from build123d import *

# Parameters (mm, degrees)
SKETCH1_R            = 2.75
SKETCH1_W            = 40
SKETCH1_H            = 15
BOSS_EXTRUDE1_DEPTH  = 10
SKETCH3_W            = 40
SKETCH3_H            = 5
BOSS_EXTRUDE2_DEPTH  = 43
CUT_EXTRUDE1_REACH   = 166.968
SKETCH4_R            = 1.75
SKETCH4_R_2          = 11
SKETCH8_W            = 4
SKETCH8_H            = 45
BOSS_EXTRUDE4_DEPTH  = 43
SKETCH11_W           = 40
SKETCH11_H           = 40
BOSS_EXTRUDE15_DEPTH = 3
FILLET3_R            = 1
FILLET6_R            = 1
FILLET7_R            = 1


with BuildPart() as part:
    # Sketch1 → Boss-Extrude1 (new body)
    with BuildSketch(Plane(origin=(0, 0, 0), x_dir=(1, 0, 0), z_dir=(0, 1, 0))):
        Polygon((51, 62.5), (51, 83.65), (99, 83.65), (99, 62.5), (150, 62.5), (150, 0), (0, 0), (0, 62.5), align=None)
        with Locations(Location((108.05464, 46, 0), (0, 0, 270))):
            Circle(SKETCH1_R, mode=Mode.SUBTRACT)
        with Locations(Location((41.87366, 46, 0), (0, 0, 270))):
            Circle(SKETCH1_R, mode=Mode.SUBTRACT)
        with Locations(Location((41.87366, 16.5, 0), (0, 0, 270))):
            Circle(SKETCH1_R, mode=Mode.SUBTRACT)
        with Locations(Location((108.05464, 16.5, 0), (0, 0, 270))):
            Circle(SKETCH1_R, mode=Mode.SUBTRACT)
        with Locations((75, 31.15)):
            Rectangle(SKETCH1_W, SKETCH1_H, mode=Mode.SUBTRACT)
    extrude(amount=BOSS_EXTRUDE1_DEPTH)

    # Sketch3 → Boss-Extrude2 (add)
    with BuildSketch(Plane(origin=(0, 10, 0), x_dir=(1, 0, 0), z_dir=(0, 1, 0))):
        with Locations((75, 41.15)):
            Rectangle(SKETCH3_W, SKETCH3_H)
    extrude(amount=BOSS_EXTRUDE2_DEPTH)

    # Sketch4 → Cut-Extrude1 (cut, up to next)
    with BuildSketch(Plane(origin=(0, 0, -43.65), x_dir=(-1, 0, 0), z_dir=(0, 0, -1)), mode=Mode.PRIVATE) as cut_extrude1_sk1:
        with Locations((-59.5, 18.25)):
            Circle(SKETCH4_R)
    cut_extrude1_tool1 = extrude(cut_extrude1_sk1.sketch, amount=-CUT_EXTRUDE1_REACH, mode=Mode.PRIVATE) & part.part
    # Sketch4 → Cut-Extrude1 (cut, up to next)
    with BuildSketch(Plane(origin=(0, 0, -43.65), x_dir=(-1, 0, 0), z_dir=(0, 0, -1)), mode=Mode.PRIVATE) as cut_extrude1_sk2:
        with Locations((-90.5, 18.25)):
            Circle(SKETCH4_R)
    cut_extrude1_tool2 = extrude(cut_extrude1_sk2.sketch, amount=-CUT_EXTRUDE1_REACH, mode=Mode.PRIVATE) & part.part
    # Sketch4 → Cut-Extrude1 (cut, up to next)
    with BuildSketch(Plane(origin=(0, 0, -43.65), x_dir=(-1, 0, 0), z_dir=(0, 0, -1)), mode=Mode.PRIVATE) as cut_extrude1_sk3:
        with Locations((-75, 33.75)):
            Circle(SKETCH4_R_2)
    cut_extrude1_tool3 = extrude(cut_extrude1_sk3.sketch, amount=-CUT_EXTRUDE1_REACH, mode=Mode.PRIVATE) & part.part
    # Sketch4 → Cut-Extrude1 (cut, up to next)
    with BuildSketch(Plane(origin=(0, 0, -43.65), x_dir=(-1, 0, 0), z_dir=(0, 0, -1)), mode=Mode.PRIVATE) as cut_extrude1_sk4:
        with Locations((-90.5, 49.25)):
            Circle(SKETCH4_R)
    cut_extrude1_tool4 = extrude(cut_extrude1_sk4.sketch, amount=-CUT_EXTRUDE1_REACH, mode=Mode.PRIVATE) & part.part
    # Sketch4 → Cut-Extrude1 (cut, up to next)
    with BuildSketch(Plane(origin=(0, 0, -43.65), x_dir=(-1, 0, 0), z_dir=(0, 0, -1)), mode=Mode.PRIVATE) as cut_extrude1_sk5:
        with Locations((-59.5, 49.25)):
            Circle(SKETCH4_R)
    cut_extrude1_tool5 = extrude(cut_extrude1_sk5.sketch, amount=-CUT_EXTRUDE1_REACH, mode=Mode.PRIVATE) & part.part
    add(cut_extrude1_tool1.solids().sort_by_distance((59.5, 18.25, -43.65))[0], mode=Mode.SUBTRACT)
    add(cut_extrude1_tool2.solids().sort_by_distance((90.5, 18.25, -43.65))[0], mode=Mode.SUBTRACT)
    add(cut_extrude1_tool3.solids().sort_by_distance((75, 33.75, -43.65))[0], mode=Mode.SUBTRACT)
    add(cut_extrude1_tool4.solids().sort_by_distance((90.5, 49.25, -43.65))[0], mode=Mode.SUBTRACT)
    add(cut_extrude1_tool5.solids().sort_by_distance((59.5, 49.25, -43.65))[0], mode=Mode.SUBTRACT)

    # Sketch8 → Boss-Extrude4 (add)
    with BuildSketch(Plane(origin=(0, 10, 0), x_dir=(1, 0, 0), z_dir=(0, 1, 0))):
        with Locations((53, 61.15)):
            Rectangle(SKETCH8_W, SKETCH8_H)
        with Locations((97, 61.15)):
            Rectangle(SKETCH8_W, SKETCH8_H)
    extrude(amount=BOSS_EXTRUDE4_DEPTH)

    # Sketch11 → Boss-Extrude15 (add)
    with BuildSketch(Plane(origin=(0, 10, 0), x_dir=(1, 0, 0), z_dir=(0, 1, 0))):
        with Locations((75, 63.65)):
            Rectangle(SKETCH11_W, SKETCH11_H)
    extrude(amount=BOSS_EXTRUDE15_DEPTH)

    # Fillet3
    fillet3_edges = [part.edges().sort_by_distance(p)[0] for p in [
        (55, 0, -31.15),
        (75, 0, -23.65),
        (95, 0, -31.15),
        (75, 0, -38.65),
        (55, 5, -38.65),
        (55, 5, -23.65),
        (95, 5, -23.65),
        (95, 5, -38.65),
    ]]
    fillet(fillet3_edges, radius=FILLET3_R)

    # Fillet6
    fillet6_edges = [part.edges().sort_by_distance(p)[0] for p in [
        (99, 10, -50.575),
        (51, 10, -50.575),
    ]]
    fillet(fillet6_edges, radius=FILLET6_R)

    # Fillet7
    fillet7_edges = [part.edges().sort_by_distance(p)[0] for p in [
        (99, 5.5, -62.5),
        (51, 5.5, -62.5),
    ]]
    fillet(fillet7_edges, radius=FILLET7_R)


solid = part.part
Input: part model. Units: mm. Frame: model coordinates. A direction names the side the tool comes from. Give positions to 0.01 mm unless a question says otherwise; leave off trailing zeros. Order: outer loops, then holes, each group sorted by start corner. A loop starts at its lowest first (then second) coordinate and runs counter-clockwise, first axis right, second up.
Q1. Section A-A on y = 49.25. Output: boundary loops of the cut face in (x, z), and give its area (3 significant figures).
Checked values:
outline: (51, -83.65) - (55, -83.65) - (55, -43.65) - (57.75, -43.65) - (57.75, -38.65) - (51, -38.65) - close; (61.25, -43.65) - (88.75, -43.65) - (88.75, -38.65) - (61.25, -38.65) - close; (92.25, -43.65) - (95, -43.65) - (95, -83.65) - (99, -83.65) - (99, -38.65) - (92.25, -38.65) - close
area: 525 mm2
Q2. Section C-C on x = 90.5. Output: boundary loops of the cut face in (y, z).
Checked values:
outline: (0, -83.65) - (13, -83.65) - (13, -43.65) - (16.5, -43.65) - (16.5, -38.65) - (1, -38.65) arc R1 ccw to (0, -39.65) - close; (0, -22.65) arc R1 ccw to (1, -23.65) - (10, -23.65) - (10, 0) - (0, 0) - close; (20, -43.65) - (47.5, -43.65) - (47.5, -38.65) - (20, -38.65) - close; (51, -43.65) - (53, -43.65) - (53, -38.65) - (51, -38.65) - close
Q3. Contact query for flat-ended pins moving along their axis: pin 1 Ø2 at (y, z) = (14.5, -65) entering from +X; pin 2 Ø1 at (x, z) = (25, -55.5) entering from +Y; pin 3 Ø5 at (x, y) = (132, 3.5) entering from -Z. Output: stop coordinate, or through.
Checked values:
pin 1: stops at x = 99
pin 2: stops at y = 10
pin 3: stops at z = -62.5
Q4. Draft query along X for faces 4 (the cylindrical face through (105.37, 4.93, -17.1)), 5 (the flat face through (51, 26, -61)), 6 (the flat face through (76, 5, 0)). Return one class per face: +X half, -X half, draft (parallel to the pull), parting line (faces both ways), or undercut.
Checked values:
face 4: undercut
face 5: -X half
face 6: draft
Q5. Set-up query: faces 1 (the flat face through (95, 5, -31)), 2 (the flat face through (66, 24, -43.65)), 3 (the flat face through (76, 10, -18)). Return all of +Z, -Z, +X, -X, +Y, -Y with unobstructed straight access to the full face (end or side cutting, diameter ignored); none if empty.
Checked values:
face 1: +Y, -Y
face 2: -Z, +Y
face 3: +Z, +Y
Q6. Ray query, probe 1 along X at (y, z) = (2.5, -46); probe 2 along X at (y, z) = (18, -41); probe 3 along Y at (x, z) = (59.5, -39.75). Return the intervals inside material, ascending.
Checked values:
probe 1: x = 0 to 39.12, 44.62 to 105.3, 110.8 to 150
probe 2: x = 51 to 57.77, 61.23 to 88.77, 92.23 to 99
probe 3: y = 0 to 16.5, 20 to 47.5, 51 to 53
Q7. Section D-D on x = 75. Output: boundary loops of the cut face in (y, z), and give its area (3 significant figures).
Checked values:
outline: (0, -83.65) - (13, -83.65) - (13, -43.65) - (22.75, -43.65) - (22.75, -38.65) - (1, -38.65) arc R1 ccw to (0, -39.65) - close; (0, -22.65) arc R1 ccw to (1, -23.65) - (10, -23.65) - (10, 0) - (0, 0) - close; (44.75, -43.65) - (53, -43.65) - (53, -38.65) - (44.75, -38.65) - close
area: 911 mm2
Q8. Section B-B on z = -16.5. Output: boundary loops of the cut face in (x, y), and give its area (3 significant figures).
Checked values:
outline: (0, 0) - (39.12, 0) - (39.12, 10) - (0, 10) - close; (44.62, 0) - (105.3, 0) - (105.3, 10) - (44.62, 10) - close; (110.8, 0) - (150, 0) - (150, 10) - (110.8, 10) - close
area: 1,390 mm2
